from build123d import *

# Parameters (mm, degrees)
ESQUISSE3_R             = 15
ENL_V_MAT_EXTRU_1_DEPTH = 10
ESQUISSE4_R             = 1.75
ENL_V_MAT_EXTRU_2_DEPTH = 10
ESQUISSE5_R             = 1.75
ENL_V_MAT_EXTRU_3_DEPTH = 10


with BuildPart() as part:
    # Esquisse1 → Révolution1 (revolve)
    with BuildSketch(Plane(origin=(0, 0, 0), x_dir=(0, 0, -1), z_dir=(1, 0, 0)), mode=Mode.PRIVATE) as r_volution1_sk:
        Polygon((101.754375518, 10), (101.754375518, 7.872703136), (102.754375518, 7.872703136), (102.754375518, 10), (113.254375518, 10), (113.254375518, 5), (115.25030387, 5), (115.25030387, 10), (120.254297163, 10), (120.254297163, 0), (0.004375518, 0), (0.004375518, 10), align=None)
    revolve(r_volution1_sk.sketch.rotate(Axis((0, 10, -0.004375518), (0, -1, 0)), 180), axis=Axis((0, 10, -0.004375518), (0, -1, 0)))

    # Esquisse3 → Enlèv. mat.-Extru.1 (cut)
    with BuildSketch(Plane(origin=(0, 10, 0), x_dir=(1, 0, 0), z_dir=(0, 1, 0))):
        with Locations(Location((0, 0, 0), (0, 0, 270))):
            Circle(ESQUISSE3_R)
    extrude(amount=-ENL_V_MAT_EXTRU_1_DEPTH, mode=Mode.SUBTRACT)

    # Esquisse4 → Enlèv. mat.-Extru.2 (cut)
    with BuildSketch(Plane.XZ):
        with Locations(Location((-25, -37, 0), (0, 0, 270))):
            Circle(ESQUISSE4_R)
        with Locations(Location((-40, 26, 0), (0, 0, 270))):
            Circle(ESQUISSE4_R)
        with Locations(Location((40, 26, 0), (0, 0, 270))):
            Circle(ESQUISSE4_R)
        with Locations(Location((30, -37, 0), (0, 0, 270))):
            Circle(ESQUISSE4_R)
    extrude(amount=-ENL_V_MAT_EXTRU_2_DEPTH, mode=Mode.SUBTRACT)

    # Esquisse5 → Enlèv. mat.-Extru.3 (cut)
    with BuildSketch(Plane.XZ):
        with Locations(Location((-65, 65, 0), (0, 0, 270))):
            Circle(ESQUISSE5_R)
        with Locations(Location((-65, -65, 0), (0, 0, 270))):
            Circle(ESQUISSE5_R)
        with Locations(Location((65, 65, 0), (0, 0, 270))):
            Circle(ESQUISSE5_R)
        with Locations(Location((65, -65, 0), (0, 0, 270))):
            Circle(ESQUISSE5_R)
    extrude(amount=-ENL_V_MAT_EXTRU_3_DEPTH, mode=Mode.SUBTRACT)


solid = part.part
The model under review builds one solid part; all positions refer to its coordinate system, in mm. A direction names the side the tool comes from. Round coordinates to 2 decimals unless told otherwise and drop trailing zeros. Loops run counter-clockwise (first coordinate to the right, second up) from the corner with the lowest first, then second, coordinate; pieces in that order, holes last. Notation, with made-up numbers: (-16.75, 31) -> (18.25, 31) arc R10 cw to (18.25, 50) -> close; hole circle Ø9 at (28.5, 44). An arc over 180 degrees is marked (long way). Return JSON: item names as keys, results as strings.
(1) Add section A-A on x = 10.5. Write out the cut boundary in (y, z) (3 decimals).
Solved:
{"outline": "(0, -119.795) -> (10, -119.795) -> (10, -114.771) -> (5, -114.771) -> (5, -112.767) -> (10, -112.767) -> (10, -102.216) -> (7.873, -102.216) -> (7.873, -101.211) -> (10, -101.211) -> (10, -10.712) -> (0, -10.712) -> close; (0, 10.712) -> (10, 10.712) -> (10, 101.202) -> (7.873, 101.202) -> (7.873, 102.208) -> (10, 102.208) -> (10, 112.758) -> (5, 112.758) -> (5, 114.762) -> (10, 114.762) -> (10, 119.786) -> (0, 119.786) -> close"}
(2) For faces 4 (the cylindrical face through (100.3, 9, -22.3)), 5 (the flat face through (115.2, 10, -8.4)), list the 3-axis set-ups (+Z, -Z, +X, -X, +Y, -Y) from which the entire face can be reached by the end or side of a thin tool; tool diameter is ignored.
Solved:
{"face 4": "+Y", "face 5": "+Z, -Z, +X, -X, +Y"}
(3) Add section B-B on z = 88. Write out the cut boundary in (x, y).
Solved:
{"outline": "(-81.95, 0) -> (81.95, 0) -> (81.95, 10) -> (74.41, 10) -> (74.41, 5) -> (71.28, 5) -> (71.28, 10) -> (53.04, 10) -> (53.04, 7.87) -> (51.07, 7.87) -> (51.07, 10) -> (-51.07, 10) -> (-51.07, 7.87) -> (-53.04, 7.87) -> (-53.04, 10) -> (-71.28, 10) -> (-71.28, 5) -> (-74.41, 5) -> (-74.41, 10) -> (-81.95, 10) -> close"}
(4) For line 1 (X direction, y = 7.75, z = -34); line 2 (X direction, y = 4.25, z = 26); line 3 (Z direction, x = -41.5, y = 9), list the stretches that pass through material, from the lowest coordinate up.
Solved:
{"line 1": "-115.34 to -110.12, -108.03 to 108.03, 110.12 to 115.34", "line 2": "-117.4 to -41.75, -38.25 to 38.25, 41.75 to 117.4", "line 3": "-112.87 to -107.52, -105.38 to -94, -92.91 to 25.1, 26.9 to 92.9, 93.99 to 105.37, 107.51 to 112.86"}
(5) The part is to be moulded in two halves that separate along Z. For faces 1 (the flat face through (25, 0, -2)), 2 (the cylindrical face through (106.682, 4.93, 55.484)), 3 (the cylindrical face through (90.27, 8.92, 46.95)), say which applies: released by +Z, released by -Z, zero draft, split by the parting line, or undercut.
Solved:
{"face 1": "zero draft", "face 2": "split by the parting line", "face 3": "undercut"}
(6) Add section C-C on x = -94. Write out the cut boundary in (y, z).
Solved:
{"outline": "(0, -75) -> (10, -75) -> (10, -66.68) -> (5, -66.68) -> (5, -63.17) -> (10, -63.17) -> (10, -41.5) -> (7.87, -41.5) -> (7.87, -38.95) -> (10, -38.95) -> (10, 38.95) -> (7.87, 38.95) -> (7.87, 41.49) -> (10, 41.49) -> (10, 63.16) -> (5, 63.16) -> (5, 66.67) -> (10, 66.67) -> (10, 74.99) -> (0, 74.99) -> close"}
(7) For pin 1 (3 mm diameter, centred on x = 65, z = -65, fed in from -Y); pin 2 (1 mm diameter, centred on y = 5, z = -54, fed in from -X); pin 3 (1.5 mm diameter, centred on y = 4, z = -74.5, fed in from +X); pin 4 (4 mm diameter, centred on y = 1.5, z = 64, fed in from -X), all flat-tipped, find the tip position at first contact; note any pin that passes through.
Solved:
{"pin 1": "through", "pin 2": "x = -107.7", "pin 3": "x = 94.98", "pin 4": "x = -103.03"}
